from build123d import *

# Parameters (mm, degrees)
F0_W     = 114.3
F0_H     = 12.7
F1_DEPTH = 3.175
F2_R     = 6.35
F3_DEPTH = 25.4
F4_R     = 3.021184
F4_R_2   = 3.02523
F4_R_3   = 3.170788
F4_R_4   = 3.070755
F4_R_5   = 3.170798
F4_R_6   = 2.930153
F4_R_7   = 2.94527
F4_R_8   = 3.090546
F4_R_9   = 3.106591
F4_R_10  = 2.82513
F4_R_11  = 3.161756
F4_R_12  = 3.03759
F4_R_13  = 3.13771
F4_R_14  = 3.0417
F4_R_15  = 3.104919
F4_R_16  = 2.990317
F4_R_17  = 3.019885
F5_DEPTH = 25.4
F6_R     = 3.185907
F6_R_2   = 2.97679
F6_R_3   = 3.061714
F7_DEPTH = 25.4
F8_R     = 3.175
F9_DEPTH = 25.4


with BuildPart() as f1:
    # F0 (on Top) → F1 (new body)
    with BuildSketch(Plane.XY):
        Polygon((31.75, -76.2), (101.6, 76.2), (-152.4, 76.2), (-82.55, -76.2), align=None)
        with Locations((-25.4, -82.55)):
            Rectangle(F0_W, F0_H)
    extrude(amount=F1_DEPTH)

    # F2 (on face) → F3 (cut)
    with BuildSketch(Plane.XY.offset(3.175)):
        with Locations((-25.4, 66.675)):
            Circle(F2_R)
    extrude(amount=-F3_DEPTH, mode=Mode.SUBTRACT)

    # F4 (on face) → F5 (cut)
    with BuildSketch(Plane(origin=(0, 0, 0), x_dir=(1, 0, 0), z_dir=(0, 0, -1))):
        with Locations((-83.284251, 51.700644)):
            Circle(F4_R)
        with Locations((-75.218096, 33.298224)):
            Circle(F4_R_2)
        with Locations((-108.495958, -3.321084)):
            Circle(F4_R_3)
        with Locations((-129.506573, -48.709944)):
            Circle(F4_R_4)
        with Locations((-131.85069, -66.695675)):
            Circle(F4_R_5)
        with Locations((-93.609944, -66.641048)):
            Circle(F4_R_6)
        with Locations((-49.322799, -66.762716)):
            Circle(F4_R_7)
        with Locations((-49.380876, -48.191752)):
            Circle(F4_R_8)
        with Locations((-62.322322, -7.321586)):
            Circle(F4_R_9)
        with Locations((-1.619848, -66.78725)):
            Circle(F4_R)
        with Locations((42.874776, -66.633321)):
            Circle(F4_R_10)
        with Locations((80.977194, -66.69376)):
            Circle(F4_R_11)
        with Locations((78.597426, -48.701756)):
            Circle(F4_R_12)
        with Locations((-1.711915, -48.14671)):
            Circle(F4_R_13)
        with Locations((11.359618, -7.188707)):
            Circle(F4_R_14)
        with Locations((57.579476, -3.127213)):
            Circle(F4_R_15)
        with Locations((24.301577, 33.58651)):
            Circle(F4_R_16)
        with Locations((32.399718, 51.890686)):
            Circle(F4_R_17)
    extrude(amount=-F5_DEPTH, mode=Mode.SUBTRACT)

    # F6 (on face) → F7 (cut)
    with BuildSketch(Plane(origin=(0, 0, 0), x_dir=(1, 0, 0), z_dir=(0, 0, -1))):
        with Locations((-69.916442, 80.901213)):
            Circle(F6_R)
        with Locations((-25.25891, 80.907866)):
            Circle(F6_R_2)
        with Locations((19.162027, 81.010833)):
            Circle(F6_R_3)
    extrude(amount=-F7_DEPTH, mode=Mode.SUBTRACT)

    # F8 (on face) → F9 (cut)
    with BuildSketch(Plane(origin=(0, 0, 0), x_dir=(1, 0, 0), z_dir=(0, 0, -1))):
        with Locations((-55.243213, 56.448877)):
            Circle(F8_R)
    extrude(amount=-F9_DEPTH, mode=Mode.SUBTRACT)


solid = f1.part
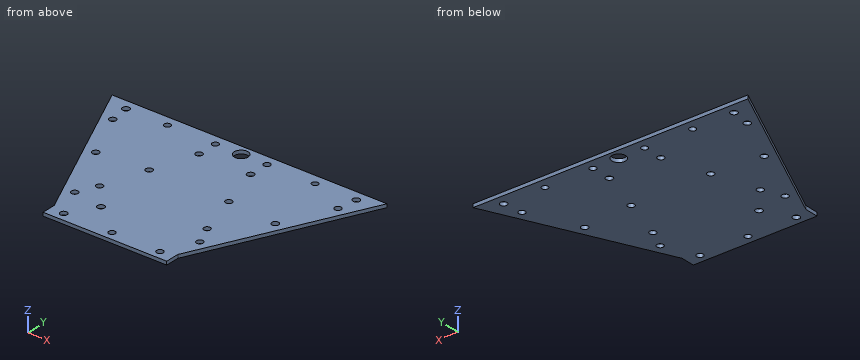
Can you work these out from the model? Positions are in its coordinate system, mm. Give positions to 0.01 mm unless a question says otherwise; leave off trailing zeros. Order: outer loops, then holes, each group sorted by start corner. A loop starts at its lowest first (then second) coordinate and runs counter-clockwise, first axis right, second up. Notation, with made-up numbers: M 78,75 L 103,75 A21 ccw 103,80 Z; hole C 36.25,36.25 d8. An arc over 180 degrees is marked long. Use one line per item in the form item = value.
Item 1: If we section it at B-B, the plane z = 2.6: Count the separate pieces of the cut face and the enclosed holes in it, and give its area (3 significant figures).
Values follow:
separate_pieces = 1
enclosed_holes = 23
area = 28,700 mm^2
Item 2: If we section it at A-A, the plane x = -25.4: Write out the boundary of the cut face in (y, z) (3 decimals).
Values follow:
outline = M -88.9,0 L -83.881,0 L -83.881,3.175 L -88.9,3.175 Z; M -77.934,0 L 60.325,0 L 60.325,3.175 L -77.934,3.175 Z; M 73.025,0 L 76.2,0 L 76.2,3.175 L 73.025,3.175 Z
Item 3: Will these pins go through, and if not, where does the flat tip stop? pin 1 Ø10 at (x, y) = (19.16, -81.01) entering from -Z; pin 2 Ø4 at (x, y) = (-55.24, -56.45) entering from +Z; pin 3 Ø1 at (y, z) = (59, 0.5) entering from +X; pin 4 Ø1 at (x, z) = (-125, 3) entering from -Y.
Values follow:
pin_1 = 0
pin_2 = through
pin_3 = 93.95
pin_4 = 15.33
Item 4: If we section it at D-D, the plane y = 38: Write out the boundary of the cut face in (x, z) (3 decimals).
Values follow:
outline = M -134.892,0 L 84.092,0 L 84.092,3.175 L -134.892,3.175 Z
Item 5: If I drill on line 1 along X through (y, z) = (-81.5, 2.3); line 2 along Y through (x, z) = (-1.5, 2.55); line 3 along X through (y, z) = (46, 1.55), over which ranges is the centre line in solid material (lowest first)? Write a range as [from, to].
Values follow:
line_1 = [-82.55, -73.05], [-66.79, -28.18], [-22.34, 16.14], [22.18, 31.75]
line_2 = [-88.9, 45.02], [51.28, 63.77], [69.81, 76.2]
line_3 = [-138.56, -130.95], [-128.06, -51.56], [-47.2, -4], [0.58, 77.21], [79.99, 87.76]
Item 6: If we section it at C-C, the plane y = 55: Write out the boundary of the cut face in (x, z) (3 decimals), and give its area (3 significant figures).
Values follow:
outline = M -142.683,0 L 91.883,0 L 91.883,3.175 L -142.683,3.175 Z
area = 745 mm^2
